from build123d import *

# Parameters (mm, degrees)
CROQUIS2_R              = 75
CROQUIS2_R_2            = 25
CROQUIS2_W              = 400
CROQUIS2_H              = 40
SALIENTE_EXTRUIR1_DEPTH = 100
CROQUIS3_W              = 60
CROQUIS3_H              = 73
CORTAR_EXTRUIR1_DEPTH   = 107


with BuildPart() as part:
    # Croquis2 → Saliente-Extruir1 (new body)
    # profile 1 of 3: a face of its own
    with BuildSketch(Plane(origin=(0, 0, 0), x_dir=(1, 0, 0), z_dir=(0, 1, 0))):
        with Locations((-200, 370)):
            Circle(CROQUIS2_R)
        with Locations(Location((-200, 370, 0), (0, 0, 270))):
            Circle(CROQUIS2_R_2, mode=Mode.SUBTRACT)
    # profile 2 of 3: a face of its own
    with BuildSketch(Plane(origin=(0, 0, 0), x_dir=(1, 0, 0), z_dir=(0, 1, 0))):
        with BuildLine():
            Line((-275, 345), (-275, 40))
            Line((-275, 40), (-200, 40))
            Line((-200, 40), (-125, 40))
            Line((-125, 40), (-125, 345))
            Line((-125, 345), (-125, 370))
            ThreePointArc((-125, 370), (-200, 295), (-275, 370))
            Line((-275, 370), (-275, 345))
        make_face()
    # profile 3 of 3: a face of its own
    with BuildSketch(Plane(origin=(0, 0, 0), x_dir=(1, 0, 0), z_dir=(0, 1, 0))):
        with Locations((-200, 20)):
            Rectangle(CROQUIS2_W, CROQUIS2_H)
    extrude(amount=SALIENTE_EXTRUIR1_DEPTH)

    # Croquis3 → Cortar-Extruir1 (cut)
    with BuildSketch(Plane.XZ):
        with Locations((-200, -376.5)):
            Rectangle(CROQUIS3_W, CROQUIS3_H)
    extrude(amount=-CORTAR_EXTRUIR1_DEPTH, mode=Mode.SUBTRACT)


solid = part.part
Design review of the part built by this model. Coordinates are the model's own, in mm. A direction names the side the tool comes from. Give positions to 0.01 mm unless a question says otherwise; leave off trailing zeros. Loops run counter-clockwise (first coordinate to the right, second up) from the corner with the lowest first, then second, coordinate; pieces in that order, holes last. Notation, with made-up numbers: (13, -20) -> (65, -20) arc R11 ccw to (65, -11) -> close; hole circle Ø2 at (35.25, 50.5). An arc over 180 degrees is marked (long way). One line per question, with ' | ' between items. Start each with the question number.
(1) For line 1 (Z direction, x = -86, y = 64); line 2 (X direction, y = 88.5, z = -216.5); line 3 (Z direction, x = -181, y = 22), list the stretches that pass through material, from the lowest coordinate up.
(2) We need section C-C (x = -361). State the section outline as (y, z) points.
(3) We need section D-D (z = -192). State the section outline as (x, y) points.
(4) We need section A-A (x = -200). State the section outline as (y, z) points, and give its area (3 significant figures).
(5) For faces 1 (the face through (-400, 49, -20)), 2 (the face through (-275, 49, -207)), 3 (the face through (-125, 49, -203)), 4 (the face through (-200, 49, -413)), list the 3-axis set-ups (+Z, -Z, +X, -X, +Y, -Y) from which the entire face can be reached by the end or side of a thin tool; tool diameter is ignored.
(6) Draft analysis for pull direction Z (two halves, no side actions). For faces 5 (the face through (-203, 100, -176)), 6 (the face through (-200, 49, -340)), 7 (the face through (-198.35, 49.3, -444.98)), 8 (the face through (-230, 49, -377)), state which applies: +Z half, -Z half, draft (parallel to the pull), parting line (faces both ways), or undercut.
(7) Insertion check: P1, Ø2, axis at y = 77, z = -69.5, coming from the +X side; P2, Ø4, axis at x = -77, y = 63.5, coming from the -Z side; P3, Ø8, axis at x = -182, y = 53.5, coming from the -Z side; P4, Ø8, axis at x = -117.5, z = -345, coming from the +Y side. Each pin has a flat end and moves straight along its axis. Give the tip position at first contact, or say it passes through.
(8) We need section B-B (y = 42.5). State the section outline as (x, z) points, and give its area (3 significant figures).
The answers:
1) line 1: z = -40 to 0 | line 2: x = -275 to -125 | line 3: z = -442.55 to -413, -340 to 0
2) outline: (0, -40) -> (100, -40) -> (100, 0) -> (0, 0) -> close
3) outline: (-275, 0) -> (-125, 0) -> (-125, 100) -> (-275, 100) -> close
4) outline: (0, -445) -> (100, -445) -> (100, -413) -> (0, -413) -> close; (0, -340) -> (100, -340) -> (100, 0) -> (0, 0) -> close | area: 37,200 mm^2
5) face 1: +Z, -Z, -X, +Y, -Y | face 2: -Z, -X, +Y, -Y | face 3: -Z, +X, +Y, -Y | face 4: +Y, -Y
6) face 5: draft | face 6: undercut | face 7: -Z half | face 8: undercut
7) P1: stops at x = -125 | P2: stops at z = -40 | P3: stops at z = -443.68 | P4: passes through
8) outline: (-400, -40) -> (-275, -40) -> (-275, -370) arc R75 ccw to (-125, -370) -> (-125, -40) -> (0, -40) -> (0, 0) -> (-400, 0) -> close; hole (-230, -413) -> (-170, -413) -> (-170, -340) -> (-230, -340) -> close | area: 70,000 mm^2
